Could you check a few things on this model? Use its own coordinates, in mm. A direction names the side the tool comes from. Give positions to 0.01 mm unless a question says otherwise; leave off trailing zeros. Write each loop counter-clockwise with the first axis right and the second up, starting at its lowest first coordinate (ties: lowest second). Pieces come first, ordered by that corner, then holes. Notation, with made-up numbers: (5.5, -17) - (36.5, -17) arc R22 cw to (36.5, 8) - close; hole circle Ø4 at (76.5, -6). An arc over 180 degrees is marked (long way). Write item = value, one per line.
from build123d import *

# Parameters (mm, degrees)
PAD_DEPTH       = 65
SKETCH052_R     = 1.625
POCKET_DEPTH    = 5
SKETCH053_R     = 2.875
POCKET001_DEPTH = 2
SKETCH054_R     = 1.35
POCKET002_DEPTH = 5
SKETCH055_W     = 20
SKETCH055_H     = 26
POCKET003_DEPTH = 2
POCKET004_DEPTH = 28
POCKET005_DEPTH = 28
PAD001_DEPTH    = 1.5
SKETCH062_W     = 12
SKETCH062_H     = 27
POCKET006_DEPTH = 1.5
CHAMFER_SIZE    = 1
FILLET_R        = 11
FILLET001_R     = 23
FILLET002_R     = 39
FILLET003_R     = 7
SKETCH063_R     = 16.544176
POCKET007_DEPTH = 5


with BuildPart() as part:
    # Sketch → Pad (new body)
    with BuildSketch(Plane.XZ):
        Polygon((0, -64), (0, 35), (-3, 35), (-3, -15), (-24, -15), (-24, -40), align=None)
    extrude(amount=PAD_DEPTH)

    # Sketch052 (on Face3 of Pad) → Pocket (cut)
    with BuildSketch(Plane(origin=(-3, 0, 0), x_dir=(0, 0, -1), z_dir=(-1, 0, 0))):
        with Locations((0, 5)):
            Circle(SKETCH052_R)
        with Locations((0, 50)):
            Circle(SKETCH052_R)
    extrude(amount=-POCKET_DEPTH, mode=Mode.SUBTRACT)

    # Sketch053 (on Face9 of Pocket) → Pocket001 (cut)
    with BuildSketch(Plane(origin=(-3, 0, 0), x_dir=(0, 0, -1), z_dir=(-1, 0, 0))):
        with Locations((0, 50)):
            Circle(SKETCH053_R)
        with Locations((0, 5)):
            Circle(SKETCH053_R)
    extrude(amount=-POCKET001_DEPTH, mode=Mode.SUBTRACT)

    # Sketch054 (on Face9 of Pocket001) → Pocket002 (cut)
    with BuildSketch(Plane(origin=(-3, 0, 0), x_dir=(0, 0, -1), z_dir=(-1, 0, 0))):
        with Locations((8.5, 60)):
            Circle(SKETCH054_R)
        with Locations((-30, 18)):
            Circle(SKETCH054_R)
    extrude(amount=-POCKET002_DEPTH, mode=Mode.SUBTRACT)

    # Sketch055 (on Face12 of Pocket002) → Pocket003 (cut)
    with BuildSketch(Plane(origin=(0, 0, -15), x_dir=(-1, 0, 0), z_dir=(0, 0, 1))):
        with Locations((13, 28)):
            Rectangle(SKETCH055_W, SKETCH055_H)
    extrude(amount=-POCKET003_DEPTH, mode=Mode.SUBTRACT)

    # Sketch056 (on Face10 of Pocket003) → Pocket004 (cut)
    with BuildSketch(Plane(origin=(-24, 0, 0), x_dir=(0, 0, -1), z_dir=(-1, 0, 0))):
        Polygon((14.286358, 43), (65, 43), (65, 13), (14.028623, 13), (14.028623, -3.205193), (140.957237, -3.205193), (140.957237, 77.307121), (13.139557, 77.307121), align=None)
    extrude(amount=-POCKET004_DEPTH, mode=Mode.SUBTRACT)

    # Sketch057 (on Face2 of Pocket004) → Pocket005 (cut)
    with BuildSketch(Plane(origin=(0, -13, 0), x_dir=(1, 0, 0), z_dir=(0, 1, 0))):
        Polygon((-22.5, 16.5), (-1.5, 16.5), (-1.5, 60.37868), (-22.5, 39.37868), align=None)
    extrude(amount=-POCKET005_DEPTH, mode=Mode.SUBTRACT)

    # Sketch061 (on Face2 of Pocket005) → Pad001 (join)
    with BuildSketch(Plane(origin=(0, -13, 0), x_dir=(1, 0, 0), z_dir=(0, 1, 0))):
        Polygon((-1.009204, 15.459926), (-23.050085, 15.459926), (-23.050085, 39.634087), (-1.009204, 61.831638), align=None)
    extrude(amount=-PAD001_DEPTH)

    # Sketch062 (on Face1 of Pad001) → Pocket006 (cut)
    with BuildSketch(Plane(origin=(0, 0, 0), x_dir=(0, 0, 1), z_dir=(1, 0, 0))):
        with Locations((-55.608883, 27.916479)):
            Rectangle(SKETCH062_W, SKETCH062_H)
    extrude(amount=-POCKET006_DEPTH, mode=Mode.SUBTRACT)

    # Chamfer
    chamfer_edges = [part.edges().sort_by_distance(p)[0] for p in [
        (0, -28, -64),
    ]]
    chamfer(chamfer_edges, length=CHAMFER_SIZE)

    # Fillet
    fillet_edges = [part.edges().sort_by_distance(p)[0] for p in [
        (-1.5, 0, -14.028623),
    ]]
    fillet(fillet_edges, radius=FILLET_R)

    # Fillet001
    fillet001_edges = [part.edges().sort_by_distance(p)[0] for p in [
        (-1.5, 0, 35),
    ]]
    fillet(fillet001_edges, radius=FILLET001_R)

    # Fillet002
    fillet002_edges = [part.edges().sort_by_distance(p)[0] for p in [
        (-1.5, -65, 35),
    ]]
    fillet(fillet002_edges, radius=FILLET002_R)

    # Fillet003
    fillet003_edges = [part.edges().sort_by_distance(p)[0] for p in [
        (-1.5, -65, -13.550953),
    ]]
    fillet(fillet003_edges, radius=FILLET003_R)

    # Sketch063 (on Face22 of Fillet003) → Pocket007 (cut)
    with BuildSketch(Plane(origin=(-3, 0, 0), x_dir=(0, 0, -1), z_dir=(-1, 0, 0))):
        with Locations((-8.708356, 28.562584)):
            Circle(SKETCH063_R)
    extrude(amount=-POCKET007_DEPTH, mode=Mode.SUBTRACT)


solid = part.part
1. If we section it at B-B, the plane y = -18: Please give me the cut outline in (x, z), and give its area (3 significant figures).
Filled sheet:
outline = (-24, -40) - (-0.71, -63.29) - (0, -63) - (0, -61.61) - (-1.5, -61.61) - (-1.5, -60.38) - (-22.5, -39.38) - (-22.5, -17) - (-23, -17) - (-23, -15) - (-24, -15) - close; (-3, -16.5) - (-1.5, -16.5) - (-1.5, -49.61) - (0, -49.61) - (0, -4.03) - (-3, -4.03) - close; (-3, 21.44) - (0, 21.44) - (0, 28.65) - (-3, 28.65) - close; (-3, 31.35) - (0, 31.35) - (0, 34.45) - (-3, 34.45) - close
area = 202 mm2
2. If we section it at A-A, the plane z = -31.5: Please give me the cut outline in (x, y), and give its area (4 significant figures).
Filled sheet:
outline = (-24, -43) - (0, -43) - (0, -13) - (-24, -13) - close; hole (-22.5, -41) - (-1.5, -41) - (-1.5, -14.5) - (-22.5, -14.5) - close
area = 163.5 mm2
3. Thinking about a two-plate mould opening in Y: for faces 1 (the face through (-23.6, -29, -15)), 2 (the face through (-1.521, -6.559, 28.084)), 3 (the face through (-0.51, -6.61, 0.21)), 4 (the face through (-12, -41, -32)), which applies, pulls with the +Y half, pulls with the -Y half, needs draft (parallel to the pull), parting line crosses it, or undercut?
Filled sheet:
face_1 = needs draft
face_2 = pulls with the +Y half
face_3 = undercut
face_4 = undercut
4. If we section it at C-C, the plane y = -5: Please give me the cut outline in (x, z) (3 decimals).
Filled sheet:
outline = (-3, -12.248) - (0, -12.248) - (0, -1.625) - (-1, -1.625) - (-1, -2.875) - (-3, -2.875) - close; (-3, 2.875) - (-1, 2.875) - (-1, 1.625) - (0, 1.625) - (0, 26.318) - (-3, 26.318) - close
5. Which directions (+Z, -Z, +X, -X, +Y, -Y) give clear straight access to the entire face, cutting with the end or side of a thin tool? Please do faces 5 (the face through (-2.01, -7.85, 0.37)), 6 (the face through (-12, -13, -34)), 7 (the face through (-2.7, -23.8, -16.5)).
Filled sheet:
face_5 = -X
face_6 = -Z, +X, -X, +Y
face_7 = none
6. I need wall thicknesses on line 1 (Y direction, x = -17.5, z = -18); line 2 (Y direction, x = -2, z = 0) (3 decimals); line 3 (X direction, y = -18, z = -30.5). Which ranges of each line are inside material? Lowest first, please.
Filled sheet:
line_1 = -43 to -41, -14.5 to -13
line_2 = -64.794 to -52.875, -47.125 to -42.629, -14.496 to -7.875, -2.125 to 0
line_3 = -24 to -22.5, -1.5 to 0
7. If we section it at D-D, the plane z = 30: Please give me the cut outline in (x, y), and give its area (3 significant figures).
Filled sheet:
outline = (-3, -45.1) - (0, -45.1) - (0, -19.35) - (-3, -19.35) - close; (-3, -16.65) - (0, -16.65) - (0, -8.68) - (-3, -8.68) - close
area = 101 mm2
8. For pin 1 (3.5 mm diameter, centred on y = -5, z = 0, fed in from -X); pin 2 (2 mm diameter, centred on x = -15, y = -40.5, fed in from +Z); pin 3 (4 mm diameter, centred on x = -18.5, z = -26.5, fed in from +Y); pin 4 (12 mm diameter, centred on x = -10.5, y = -51.5, fed in from +Z), each with a flat end and sliding along its axis, tell me the tip position at first contact or that it passes through.
Filled sheet:
pin_1 = -1
pin_2 = -15
pin_3 = -13
pin_4 = through
